from build123d import *

# Parameters (mm, degrees)
SKETCH1_R           = 5.354341082
BOSS_EXTRUDE1_DEPTH = 3.81
FILLET1_R           = 2.54
CUT_EXTRUDE1_DEPTH  = 2.794
SKETCH3_R           = 1.69700591
BOSS_EXTRUDE2_DEPTH = 16.256


with BuildPart() as part:
    # Sketch1 → Boss-Extrude1 (new body)
    with BuildSketch(Plane.XY):
        Circle(SKETCH1_R)
    extrude(amount=BOSS_EXTRUDE1_DEPTH)

    # Fillet1
    fillet1_edges = [part.edges().sort_by_distance(p)[0] for p in [
        (-5.354341082, 0, 3.81),
    ]]
    fillet(fillet1_edges, radius=FILLET1_R)

    # Sketch2 → Cut-Extrude1 (cut)
    with BuildSketch(Plane.XY.offset(3.81)):
        Polygon((0, 1.998303372), (-1.730581485, 0.999151686), (-1.730581485, -0.999151686), (0, -1.998303372), (1.730581485, -0.999151686), (1.730581485, 0.999151686), align=None)
    extrude(amount=-CUT_EXTRUDE1_DEPTH, mode=Mode.SUBTRACT)

    # Sketch3 → Boss-Extrude2 (add)
    with BuildSketch(Plane(origin=(0, 0, 0), x_dir=(-1, 0, 0), z_dir=(0, 0, -1))):
        Circle(SKETCH3_R)
    extrude(amount=BOSS_EXTRUDE2_DEPTH)


solid = part.part
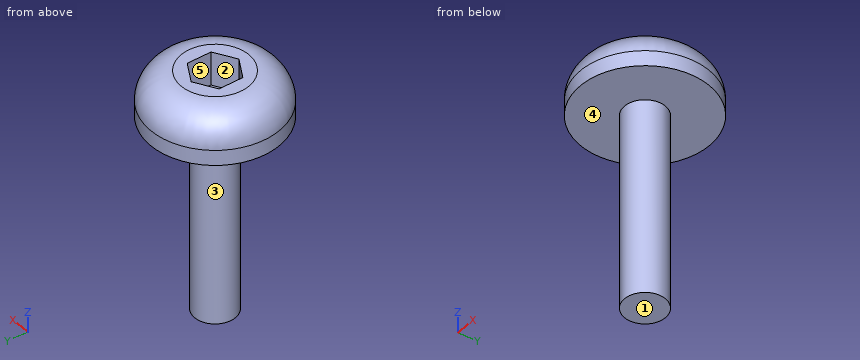
Work out the finished part from the listing and answer in its coordinate system (mm). Face numbers are marked on the shaded views. A direction names the side the tool comes from. Coordinates: 2 decimals unless noted, no trailing zeros. Order: outer loops, then holes, each group sorted by start corner. A loop starts at its lowest first (then second) coordinate and runs counter-clockwise, first axis right, second up. Notation, with made-up numbers: (73.5, 16) - (85.5, 16) arc R20 ccw to (85.5, 28) - close; hole circle Ø11 at (74.5, -7.75). An arc over 180 degrees is marked (long way). Put each result on its own line as item: value. Start each with the question number.
1) Find section B-B (z = -7.5). Give the vertices of the cut face in (x, y).
2) Find the intervals of material crossed by line 1 (Z direction, x = -0.5, y = 0); line 2 (Z direction, x = 0.75, y = 2.25); line 3 (X direction, y = 1, z = -15), in increasing order. Write a range as from..to.
3) Flat-ended cylindrical pins translate along their axes: pin 1 (1.6 mm diameter, centred on y = 0, z = 2, fed in from -X); pin 2 (4 mm diameter, centred on x = 2.5, z = -10, fed in from +Y); pin 3 (3 mm diameter, centred on x = 2, z = 1.5, fed in from -Y); pin 4 (4 mm diameter, centred on x = 3.5, y = 3.5, fed in from -Z). Find the tip coordinate at first contact, or state that the pin passes through.
4) Find section A-A (y = 0). Give the vertices of the cut face in (x, z), plus the area to 3 significant figures.
5) For a pull along X with two mould halves and no side action, classify the marked faces 1, 2 and 3 as released by +X, released by -X, zero draft, split by the parting line, or undercut.
6) For the marked faces 4 and 5, determine the directions among +Z, -Z, +X, -X, +Y, -Y from which every point of the face is accessible in a straight line to the end or side of a thin tool.
Results list:
1. outline: circle Ø3.39 at (0, 0)
2. line 1: z = -16.26..1.02
2. line 2: z = 0..3.81
2. line 3: x = -1.37..1.37
3. pin 1: stops at x = -5.35
3. pin 2: stops at y = 1.62
3. pin 3: stops at y = -5.33
3. pin 4: stops at z = 0
4. outline: (-5.35, 0) - (-1.7, 0) - (-1.7, -16.26) - (1.7, -16.26) - (1.7, 0) - (5.35, 0) - (5.35, 1.27) arc R2.54 ccw to (2.81, 3.81) - (1.73, 3.81) - (1.73, 1.02) - (-1.73, 1.02) - (-1.73, 3.81) - (-2.81, 3.81) arc R2.54 ccw to (-5.35, 1.27) - close
4. area: 83.5 mm^2
5. face 1: zero draft
5. face 2: undercut
5. face 3: split by the parting line
6. face 4: -Z
6. face 5: +Z
